from build123d import *

# Parameters (mm, degrees)
F1_DEPTH = 15
F3_DEPTH = 85
F4_R     = 9.2721053172
F5_DEPTH = 100.001


with BuildPart() as f1:
    # F0 (on Front) → F1 (new body)
    with BuildSketch(Plane.XZ):
        Polygon((-100, 0), (0, 0), (-60, 85), (-100, 85), align=None)
    extrude(amount=F1_DEPTH)

    # F2 (on face) → F3 (join)
    with BuildSketch(Plane.XZ.offset(15)):
        Polygon((-65, 75), (-100, 75), (-100, 0), (-12.0588235294, 0), align=None)
    extrude(amount=F3_DEPTH)

    # F4 (on face) → F5 (cut, through all)
    with BuildSketch(Plane(origin=(-100, 0, 0), x_dir=(0, -1, 0), z_dir=(-1, 0, 0))):
        with Locations((57.5, 37.5)):
            Circle(F4_R)
    extrude(amount=-F5_DEPTH, mode=Mode.SUBTRACT)


solid = f1.part
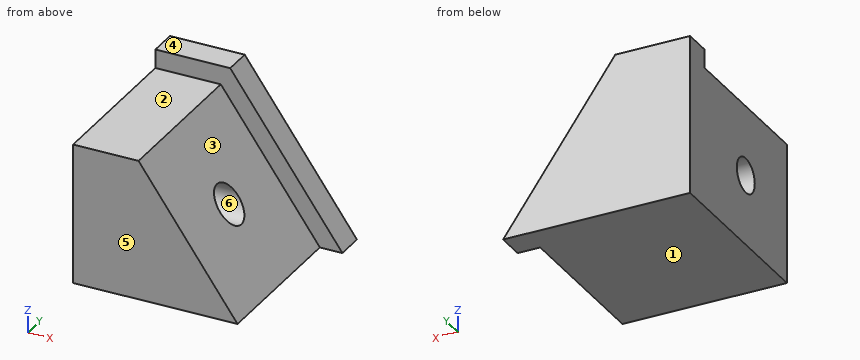
Design review of the part built by this model. Coordinates are the model's own, in mm. Face numbers are marked on the shaded views. A direction names the side the tool comes from. Round coordinates to 2 decimals unless told otherwise and drop trailing zeros. Loops run counter-clockwise (first coordinate to the right, second up) from the corner with the lowest first, then second, coordinate; pieces in that order, holes last. Notation, with made-up numbers: (-35.75, -25) - (11.25, -25) arc R12 cw to (11.25, -20) - close; hole circle Ø3 at (84.5, 55). An arc over 180 degrees is marked (long way). One line per item, written item: value. Start each with the question number.
1) Draft analysis for pull direction Z (two halves, no side actions). For the marked faces 4, 5 and 6, state which applies: +Z half, -Z half, draft (parallel to the pull), parting line (faces both ways), or undercut.
2) To check wall thickness, follow L1, parallel to Y at x = -84, z = 37.5; L2, parallel to Z at x = -83, y = -57.5; L3, parallel to Y at x = -22.5, z = 23. State the ranges of each line that lie inside material, in increasing order. Write a range as from..to.
3) For the marked faces 1, 2 and 3, list the 3-axis set-ups (+Z, -Z, +X, -X, +Y, -Y) from which the entire face can be reached by the end or side of a thin tool; tool diameter is ignored.
4) Consider section B-B on y = -63.5. Give the boundary of the cut face in (x, z), then the cut area to 3 significant figures.
5) Consider section C-C on z = 37.5. Give the boundary of the cut face in (x, y), then the cut area to 3 significant figures.
6) Consider section D-D on y = -32.5. Give the boundary of the cut face in (x, z), then the cut area to 3 significant figures.
7) Insertion check: pin 1 Ø2 at (y, z) = (-60.5, 15) entering from +X; pin 2 Ø10 at (x, y) = (-88.5, -38) entering from -Z; pin 3 Ø5 at (y, z) = (-45.5, 16) entering from +X; pin 4 Ø4 at (y, z) = (-64.5, 40.5) entering from +X. Each pin has a flat end and moves straight along its axis. Give the tip position at first contact, or say it passes through.
8) Consider section A-A on x = -92.5. Give the boundary of the cut face in (y, z).
Reported:
1. face 4: +Z half
1. face 5: draft
1. face 6: undercut
2. L1: y = -100..-66.77, -48.23..0
2. L2: z = 0..28.23, 46.77..75
2. L3: y = -15..0
3. face 1: -Z, +X, -X, +Y, -Y
3. face 2: +Z, +X, -X, -Y
3. face 3: +Z, +X, -Y
4. outline: (-100, 0) - (-12.06, 0) - (-33.54, 30.43) - (-100, 30.43) - close; (-100, 44.57) - (-43.52, 44.57) - (-65, 75) - (-100, 75) - close
4. area: 3,740 mm^2
5. outline: (-100, -100) - (-38.53, -100) - (-38.53, -66.77) - (-100, -66.77) - close; (-100, -48.23) - (-38.53, -48.23) - (-38.53, -15) - (-26.47, -15) - (-26.47, 0) - (-100, 0) - close
5. area: 5,190 mm^2
6. outline: (-100, 0) - (-12.06, 0) - (-65, 75) - (-100, 75) - close
6. area: 4,610 mm^2
7. pin 1: stops at x = -21.94
7. pin 2: stops at z = 0
7. pin 3: stops at x = -21.59
7. pin 4: stops at x = -40.28
8. outline: (-100, 0) - (0, 0) - (0, 85) - (-15, 85) - (-15, 75) - (-100, 75) - close; hole circle Ø18.54 at (-57.5, 37.5)
